```python
from build123d import *

# Parameters (mm, degrees)
SKIZZE1_R                       = 9
AUFSATZ_LINEAR_AUSTRAGEN1_DEPTH = 22
SKIZZE2_R                       = 6
SCHNITT_LINEAR_AUSTRAGEN1_DEPTH = 26.416530054
LINEARES_MUSTER1_COUNT          = 2
LINEARES_MUSTER1_PITCH          = 16
LINEARES_MUSTER2_COUNT          = 2
LINEARES_MUSTER2_PITCH          = 16


with BuildPart() as part:
    # Skizze1 → Aufsatz-Linear austragen1 (new body)
    with BuildSketch(Plane.XY):
        Circle(SKIZZE1_R)
    extrude(amount=AUFSATZ_LINEAR_AUSTRAGEN1_DEPTH)

    # Skizze2 → Schnitt-Linear austragen1 (cut, through all)
    with BuildSketch(Plane.XY.offset(22)):
        Circle(SKIZZE2_R)
    extrude(amount=-SCHNITT_LINEAR_AUSTRAGEN1_DEPTH, mode=Mode.SUBTRACT)

    # Skizze4 → M2 Gewindebohrung1 (revolve, cut)
    with BuildSketch(Plane(origin=(9, 0, 4), x_dir=(0, 0, -1), z_dir=(0, 1, 0))):
        Polygon((0, 0), (0, 6.480688495), (0.8, 6), (0.8, 0), align=None)
    m2_gewindebohrung1 = revolve(axis=Axis((15.35, 0, 4), (-1, 0, 0)), mode=Mode.SUBTRACT)

    # Skizze6 → M2 Gewindebohrung2 (revolve, cut)
    with BuildSketch(Plane(origin=(0, 9, 4), x_dir=(0, 0, 1), z_dir=(1, 0, 0))):
        Polygon((0, 0), (0, 6.480688495), (0.8, 6), (0.8, 0), align=None)
    m2_gewindebohrung2 = revolve(axis=Axis((0, 15.35, 4), (0, -1, 0)), mode=Mode.SUBTRACT)

    # Lineares Muster1: M2 Gewindebohrung1 ×2
    with Locations(*[(0, 0, i * LINEARES_MUSTER1_PITCH) for i in range(1, LINEARES_MUSTER1_COUNT)]):
        add(m2_gewindebohrung1, mode=Mode.SUBTRACT)

    # Lineares Muster2: M2 Gewindebohrung2 ×2
    with Locations(*[(0, 0, i * LINEARES_MUSTER2_PITCH) for i in range(1, LINEARES_MUSTER2_COUNT)]):
        add(m2_gewindebohrung2, mode=Mode.SUBTRACT)


solid = part.part
```
Verification items for the finished model (mm, model axes). A direction names the side the tool comes from. Coordinates: 2 decimals unless noted, no trailing zeros. Order: outer loops, then holes, each group sorted by start corner. A loop starts at its lowest first (then second) coordinate and runs counter-clockwise, first axis right, second up. Notation, with made-up numbers: (-35.5, 36.25) - (-30.5, 36.25) arc R13 cw to (-30.5, 42.25) - close; hole circle Ø9 at (-3.5, -9). An arc over 180 degrees is marked (long way). Return JSON: item names as keys, results as strings.
(1) Access from +Z, -Z, +X, -X, +Y, -Y to the whole of each face (thin tool, end or side, straight path). Record for faces 4 (the cylindrical face through (7.49, 0.78, 20.17)), 5 (the cylindrical face through (-1.172, 8.923, 10.846)), 6 (the cylindrical face through (0, 7.5, 3.2)).
Filled sheet:
{"face 4": "+X", "face 5": "+Z, -Z", "face 6": "+Y"}
(2) Section check D-D, the plane y = -0.5. Record the cut outline in (x, z), and give its area (3 significant figures).
Filled sheet:
{"outline": "(-8.99, 0) - (-5.98, 0) - (-5.98, 22) - (-8.99, 22) - close; (5.98, 0) - (8.99, 0) - (8.99, 3.38) - (5.98, 3.38) - close; (5.98, 4.62) - (8.99, 4.62) - (8.99, 19.38) - (5.98, 19.38) - close; (5.98, 20.62) - (8.99, 20.62) - (8.99, 22) - (5.98, 22) - close", "area": "125 mm^2"}
(3) Section check C-C, the plane y = 4.25. Record the cut outline in (x, z), and give its area (3 significant figures).
Filled sheet:
{"outline": "(-7.93, 0) - (-4.24, 0) - (-4.24, 22) - (-7.93, 22) - close; (4.24, 0) - (7.93, 0) - (7.93, 22) - (4.24, 22) - close", "area": "163 mm^2"}
(4) Section check B-B, the plane z = 20.25. Record the cut outline in (x, y), and give its area (3 significant figures).
Filled sheet:
{"outline": "(-0.76, 5.95) - (-0.76, 8.97) arc R9 ccw (long way) to (8.97, -0.76) - (5.95, -0.76) arc R6 cw (long way) to start; (0.76, 5.95) arc R6 cw to (5.95, 0.76) - (8.97, 0.76) arc R9 ccw to (0.76, 8.97) - close", "area": "132 mm^2"}
(5) Section check A-A, the plane x = 0. Record the cut outline in (y, z), and give its area (3 significant figures).
Filled sheet:
{"outline": "(-9, 0) - (-6, 0) - (-6, 22) - (-9, 22) - close; (6, 0) - (9, 0) - (9, 3.2) - (6, 3.2) - close; (6, 4.8) - (9, 4.8) - (9, 19.2) - (6, 19.2) - close; (6, 20.8) - (9, 20.8) - (9, 22) - (6, 22) - close", "area": "122 mm^2"}
(6) Thickness scan on line 1 along Z through (x, y) = (8.3, 0); line 2 along Y through (x, z) = (-5.5, 6.5); line 3 along X through (y, z) = (7.05, 20). Record the ranges inside material, lowest first.
Filled sheet:
{"line 1": "z = 0 to 3.2, 4.8 to 19.2, 20.8 to 22", "line 2": "y = -7.12 to -2.4, 2.4 to 7.12", "line 3": "x = -5.59 to -0.8, 0.8 to 5.59"}
(7) Mould release check, pull along Z, two halves, no side actions. Record for faces 1 (the flat face through (2, -6, 22)), 2 (the cylindrical face through (7.5, 0, 4.8)), 3 (the flat face through (2, -6, 0)): pulls with the +Z half, pulls with the -Z half, needs draft (parallel to the pull), parting line crosses it, or undercut.
Filled sheet:
{"face 1": "pulls with the +Z half", "face 2": "undercut", "face 3": "pulls with the -Z half"}
(8) Go/stop test with flat-tipped pins: pin 1 (5 mm diameter, centred on y = 4, z = 18, fed in from +X); pin 2 (1.4 mm diameter, centred on x = 0, z = 20, fed in from +Y); pin 3 (6 mm diameter, centred on y = 3.5, z = 16, fed in from +X). Record where each tip stops, or that it passes through.
Filled sheet:
{"pin 1": "stops at x = 8.87", "pin 2": "stops at y = -5.96", "pin 3": "stops at x = 8.99"}
